Part model, mm, in its own coordinate system. Face numbers are marked on the shaded views. A direction names the side the tool comes from. Round coordinates to 2 decimals unless told otherwise and drop trailing zeros. Order: outer loops, then holes, each group sorted by start corner. A loop starts at its lowest first (then second) coordinate and runs counter-clockwise, first axis right, second up. Notation, with made-up numbers: (57.25, -8.5) -> (72.25, -8.5) arc R17 cw to (72.25, 11.5) -> close; hole circle Ø8 at (-26, 50.25). An arc over 180 degrees is marked (long way). Answer as a JSON object with one key per item and string values. Group by question number.
```python
from build123d import *

# Parameters (mm, degrees)
SKETCH1_W           = 79.5
SKETCH1_H           = 49
BOSS_EXTRUDE1_DEPTH = 15
SKETCH2_W           = 64
SKETCH2_H           = 34.5
CUT_EXTRUDE1_DEPTH  = 13
SKETCH3_W           = 75.5
SKETCH3_H           = 45
CUT_EXTRUDE2_DEPTH  = 1
CUT_EXTRUDE3_REACH  = 96.585
SKETCH5_W           = 10.77
SKETCH5_H           = 1
LIP1_START          = -48
LIP1_DEPTH          = 1
LIP1_START_2        = -2
LIP1_2_DEPTH        = 1
LIP1_START_3        = -47
LIP1_3_DEPTH        = 32.35
LIP1_START_4        = -14.65
LIP1_4_DEPTH        = 12.65
LIP1_START_5        = -3.88
LIP1_5_DEPTH        = 1.88
LIP1_6_DEPTH        = 79


with BuildPart() as part:
    # Sketch1 → Boss-Extrude1 (new body)
    with BuildSketch(Plane(origin=(0, 0, 0), x_dir=(1, 0, 0), z_dir=(0, 1, 0))):
        with Locations((39.75, 24.5)):
            Rectangle(SKETCH1_W, SKETCH1_H)
    extrude(amount=BOSS_EXTRUDE1_DEPTH)

    # Sketch2 → Cut-Extrude1 (cut)
    with BuildSketch(Plane(origin=(0, 15, 0), x_dir=(1, 0, 0), z_dir=(0, 1, 0))):
        with Locations((39.5, 23.59)):
            Rectangle(SKETCH2_W, SKETCH2_H)
    extrude(amount=-CUT_EXTRUDE1_DEPTH, mode=Mode.SUBTRACT)

    # Sketch3 → Cut-Extrude2 (cut)
    with BuildSketch(Plane(origin=(0, 15, 0), x_dir=(1, 0, 0), z_dir=(0, 1, 0))):
        with Locations((39.75, 24.5)):
            Rectangle(SKETCH3_W, SKETCH3_H)
    extrude(amount=-CUT_EXTRUDE2_DEPTH, mode=Mode.SUBTRACT)

    # Sketch5 → Cut-Extrude3 (cut, up to next)
    with BuildSketch(Plane(origin=(79.5, 0, 0), x_dir=(0, 0, -1), z_dir=(1, 0, 0)), mode=Mode.PRIVATE) as cut_extrude3_sk1:
        with Locations((9.265, 14.5)):
            Rectangle(SKETCH5_W, SKETCH5_H)
    cut_extrude3_tool1 = extrude(cut_extrude3_sk1.sketch, amount=-CUT_EXTRUDE3_REACH, mode=Mode.PRIVATE) & part.part
    add(cut_extrude3_tool1.solids().sort_by_distance((79.5, 14.5, -9.265))[0], mode=Mode.SUBTRACT)

    # Lip1: read off the stored shape, not the designer's step
    # Lip1 outline → Lip1 (add)
    with BuildSketch(Plane.XY.offset(LIP1_START)):
        Polygon((78.5, 15), (78.395184441, 17), (1.104815559, 17), (1, 15), align=None)
    extrude(amount=LIP1_DEPTH)

    # Lip1 2 outline → Lip1 2 (add)
    with BuildSketch(Plane.XY.offset(LIP1_START_2)):
        Polygon((78.5, 15), (78.395184441, 17), (1.104815559, 17), (1, 15), align=None)
    extrude(amount=LIP1_2_DEPTH)

    # Lip1 3 outline → Lip1 3 (add)
    with BuildSketch(Plane.XY.offset(LIP1_START_3)):
        Polygon((77.5, 17), (77.5, 15), (78.5, 15), (78.395184441, 17), align=None)
        Polygon((1, 15), (2, 15), (2, 17), (1.104815559, 17), align=None)
    extrude(amount=LIP1_3_DEPTH)

    # Lip1 4 outline → Lip1 4 (add)
    with BuildSketch(Plane.XY.offset(LIP1_START_4)):
        Polygon((1, 15), (2, 15), (2, 17), (1.104815559, 17), align=None)
    extrude(amount=LIP1_4_DEPTH)

    # Lip1 5 outline → Lip1 5 (add)
    with BuildSketch(Plane.XY.offset(LIP1_START_5)):
        Polygon((77.5, 17), (77.5, 15), (78.5, 15), (78.395184441, 17), align=None)
    extrude(amount=LIP1_5_DEPTH)

    # Lip1 6 outline → Lip1 6 (cut)
    with BuildSketch(Plane.YZ):
        Polygon((17, -48), (17, -47.895184441), (15, -48), align=None)
        Polygon((15, -1), (17, -1.104815559), (17, -1), align=None)
    extrude(amount=LIP1_6_DEPTH, mode=Mode.SUBTRACT)


solid = part.part
```
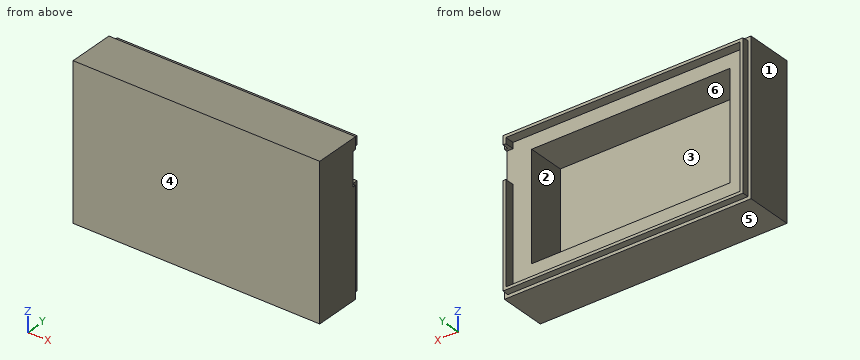
Q1. Drop flat-ended pins along their axis: pin 1 Ø1.5 at (x, z) = (31, -20) entering from +Y; pin 2 Ø1.5 at (x, z) = (34.5, -42) entering from +Y; pin 3 Ø0.9 at (x, y) = (21.5, 15.5) entering from -Z. Give the stop position or say it passes through.
Q2. Band-saw the part on A-A (y = 12.25). List the corners of the cut face in (x, z), plus the area to 3 significant figures.
Q3. Which spindle directions (+Z, -Z, +X, -X, +Y, -Y) get a long thin tool onto all of the face, cutting with end or side? Do the marked faces 1 and 2. Say none if no direction does.
Q4. Band-saw the part on B-B (x = 40). List the corners of the cut face in (y, z).
Q5. Band-saw the part on C-C (z = -33.5). List the corners of the cut face in (x, y), plus the area to 3 significant figures.
Q6. Band-saw the part on D-D (z = -13). List the corners of the cut face in (x, y), plus the area to 3 significant figures.
Q7. Two-plate mould, pull along Z, no slides. Class the marked faces 3, 4, 5 and 6: +Z half, -Z half, draft (parallel to the pull), parting line (faces both ways), or undercut.
Q8. Wall check: line 1 (Z direction, x = 67, y = 3); line 2 (X direction, y = 4, z = -14); line 3 (X direction, y = 14.75, z = -45.5). Give the ranges that are in metal, low to high. Write a range as [from, to].
Completed:
{
 "1": {"pin 1": "y = 2", "pin 2": "y = 14", "pin 3": "z = -48"},
 "2": {"outline": "(0, -49) -> (79.5, -49) -> (79.5, 0) -> (0, 0) -> close; hole (7.5, -40.84) -> (71.5, -40.84) -> (71.5, -6.34) -> (7.5, -6.34) -> close", "area": "1,690 mm2"},
 "3": {"face 1": "+Z, -Z, -X, +Y, -Y", "face 2": "+Y"},
 "4": {"outline": "(0, -49) -> (15, -49) -> (15, -48) -> (17, -47.9) -> (17, -47) -> (14, -47) -> (14, -40.84) -> (2, -40.84) -> (2, -6.34) -> (14, -6.34) -> (14, -2) -> (17, -2) -> (17, -1.1) -> (15, -1) -> (15, 0) -> (0, 0) -> close"},
 "5": {"outline": "(0, 0) -> (79.5, 0) -> (79.5, 15) -> (78.5, 15) -> (78.4, 17) -> (77.5, 17) -> (77.5, 14) -> (71.5, 14) -> (71.5, 2) -> (7.5, 2) -> (7.5, 14) -> (2, 14) -> (2, 17) -> (1.1, 17) -> (1, 15) -> (0, 15) -> close", "area": "353 mm2"},
 "6": {"outline": "(0, 0) -> (79.5, 0) -> (79.5, 14) -> (71.5, 14) -> (71.5, 2) -> (7.5, 2) -> (7.5, 14) -> (2, 14) -> (2, 17) -> (1.1, 17) -> (1, 15) -> (0, 15) -> close", "area": "349 mm2"},
 "7": {"face 3": "undercut", "face 4": "draft", "face 5": "-Z half", "face 6": "undercut"},
 "8": {"line 1": "[-49, -40.84], [-6.34, 0]", "line 2": "[0, 7.5], [71.5, 79.5]", "line 3": "[0, 2], [77.5, 79.5]"}
}
